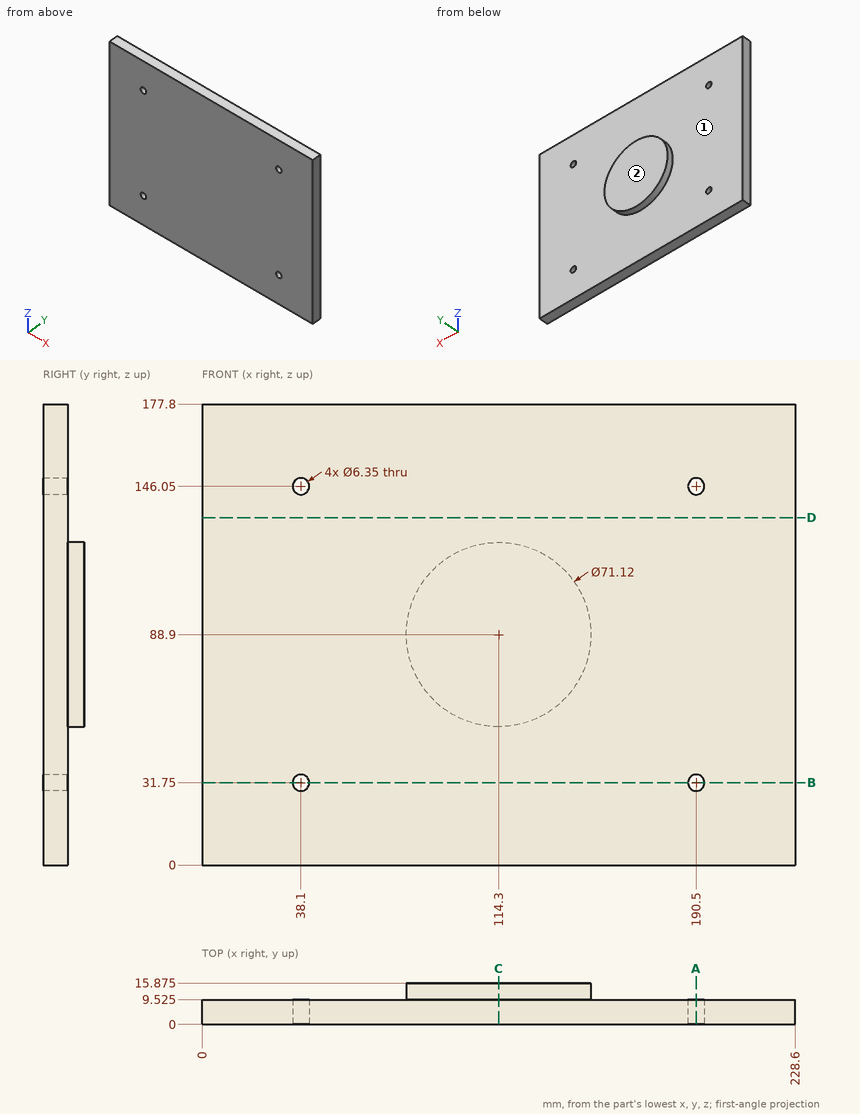
Here's the drawing with two shaded views (mm, measured from the low corner). I have some questions. A direction names the side the tool comes from. Round coordinates to 2 decimals unless told otherwise and drop trailing zeros. Order: outer loops, then holes, each group sorted by start corner. A loop starts at its lowest first (then second) coordinate and runs counter-clockwise, first axis right, second up. Notation, with made-up numbers: (-22.5, 71.25) -> (-17.5, 71.25) arc R8 ccw to (-17.5, 79.25) -> close; hole circle Ø1 at (-1, -6). An arc over 180 degrees is marked (long way). Return JSON: item names as keys, results as strings.
Q1. For pin 1 Ø10 at (x, z) = (38.1, 146.05) entering from +Y (3 decimals), with a flat end and sliding along its axis, tell me the tip position at first contact or that it passes through.
Filled sheet:
{"pin 1": "stops at y = 9.525"}
Q2. If we section it at D-D on z = 134: List the corners of the cut face in (x, y) for me (3 decimals).
Filled sheet:
{"outline": "(0, 0) -> (228.6, 0) -> (228.6, 9.525) -> (0, 9.525) -> close"}
Q3. If we section it at A-A on x = 190.5: List the corners of the cut face in (y, z) for me (3 decimals).
Filled sheet:
{"outline": "(0, 0) -> (9.525, 0) -> (9.525, 28.575) -> (0, 28.575) -> close; (0, 34.925) -> (9.525, 34.925) -> (9.525, 142.875) -> (0, 142.875) -> close; (0, 149.225) -> (9.525, 149.225) -> (9.525, 177.8) -> (0, 177.8) -> close"}
Q4. I need wall thicknesses on line 1 along Z through (x, y) = (38.1, 3.5) (3 decimals); line 2 along X through (y, z) = (6.5, 146.05) (3 decimals); line 3 along X through (y, z) = (8, 29.5). Which ranges of each line are inside material? Lowest first, please. Write a range as from..to.
Filled sheet:
{"line 1": "z = 0..28.575, 34.925..142.875, 149.225..177.8", "line 2": "x = 0..34.925, 41.275..187.325, 193.675..228.6", "line 3": "x = 0..35.86, 40.34..188.26, 192.74..228.6"}
Q5. If we section it at C-C on x = 114.3: List the corners of the cut face in (y, z) for me (3 decimals), plus the area to 3 significant figures.
Filled sheet:
{"outline": "(0, 0) -> (9.525, 0) -> (9.525, 53.34) -> (15.875, 53.34) -> (15.875, 124.46) -> (9.525, 124.46) -> (9.525, 177.8) -> (0, 177.8) -> close", "area": "2,150 mm^2"}
Q6. Which directions (+Z, -Z, +X, -X, +Y, -Y) give clear straight access to the entire face, cutting with the end or side of a thin tool? Please do the marked faces 1 and 2.
Filled sheet:
{"face 1": "+Y", "face 2": "+Z, -Z, +X, -X, +Y"}
Q7. If we section it at B-B on z = 31.75: List the corners of the cut face in (x, y) for me (3 decimals).
Filled sheet:
{"outline": "(0, 0) -> (34.925, 0) -> (34.925, 9.525) -> (0, 9.525) -> close; (41.275, 0) -> (187.325, 0) -> (187.325, 9.525) -> (41.275, 9.525) -> close; (193.675, 0) -> (228.6, 0) -> (228.6, 9.525) -> (193.675, 9.525) -> close"}
